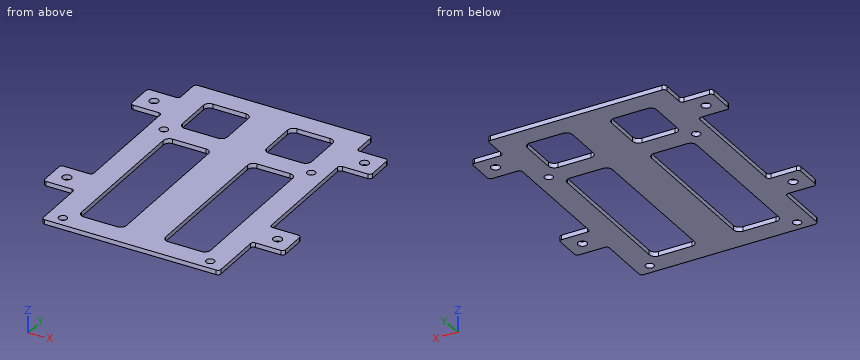
```python
from build123d import *

# Parameters (mm, degrees)
MODEL_R         = 1.375
MODEL_R_2       = 1.5
EXTRUDE_1_DEPTH = 1.5


with BuildPart() as part:
    # Model → Бобышка-Вытянуть1 (new body)
    with BuildSketch(Plane.XY):
        with BuildLine():
            ThreePointArc((-28.5, 7.535944945), (-29.207106781, 7.243051726), (-29.5, 6.535944945))
            Line((-29.5, 6.535944945), (-29.5, -0.464055055))
            ThreePointArc((-29.5, -0.464055055), (-29.792893219, -1.171161836), (-30.5, -1.464055055))
            Line((-30.5, -1.464055055), (-39, -1.464055055))
            ThreePointArc((-39, -1.464055055), (-39.707106781, -1.756948274), (-40, -2.464055055))
            Line((-40, -2.464055055), (-40, -10.464055055))
            ThreePointArc((-40, -10.464055055), (-39.707106781, -11.171161836), (-39, -11.464055055))
            Line((-39, -11.464055055), (-30.5, -11.464055055))
            ThreePointArc((-30.5, -11.464055055), (-29.792893219, -11.756948274), (-29.5, -12.464055055))
            Line((-29.5, -12.464055055), (-29.5, -50.464055055))
            ThreePointArc((-29.5, -50.464055055), (-29.792893219, -51.171161836), (-30.5, -51.464055055))
            Line((-30.5, -51.464055055), (-39, -51.464055055))
            ThreePointArc((-39, -51.464055055), (-39.707106781, -51.756948274), (-40, -52.464055055))
            Line((-40, -52.464055055), (-40, -60.464055055))
            ThreePointArc((-40, -60.464055055), (-39.707106781, -61.171161836), (-39, -61.464055055))
            Line((-39, -61.464055055), (-30.5, -61.464055055))
            ThreePointArc((-30.5, -61.464055055), (-29.792893219, -61.756948274), (-29.5, -62.464055055))
            Line((-29.5, -62.464055055), (-29.5, -79.464055055))
            ThreePointArc((-29.5, -79.464055055), (-29.207106781, -80.171161836), (-28.5, -80.464055055))
            Line((-28.5, -80.464055055), (28.5, -80.464055055))
            ThreePointArc((28.5, -80.464055055), (29.207106781, -80.171161836), (29.5, -79.464055055))
            Line((29.5, -79.464055055), (29.5, -62.464055055))
            ThreePointArc((29.5, -62.464055055), (29.792893219, -61.756948274), (30.5, -61.464055055))
            Line((30.5, -61.464055055), (39, -61.464055055))
            ThreePointArc((39, -61.464055055), (39.707106781, -61.171161836), (40, -60.464055055))
            Line((40, -60.464055055), (40, -52.464055055))
            ThreePointArc((40, -52.464055055), (39.707106781, -51.756948274), (39, -51.464055055))
            Line((39, -51.464055055), (30.5, -51.464055055))
            ThreePointArc((30.5, -51.464055055), (29.792893219, -51.171161836), (29.5, -50.464055055))
            Line((29.5, -50.464055055), (29.5, -12.464055055))
            ThreePointArc((29.5, -12.464055055), (29.792893219, -11.756948274), (30.5, -11.464055055))
            Line((30.5, -11.464055055), (39, -11.464055055))
            ThreePointArc((39, -11.464055055), (39.707106781, -11.171161836), (40, -10.464055055))
            Line((40, -10.464055055), (40, -2.464055055))
            ThreePointArc((40, -2.464055055), (39.707106781, -1.756948274), (39, -1.464055055))
            Line((39, -1.464055055), (30.5, -1.464055055))
            ThreePointArc((30.5, -1.464055055), (29.792893219, -1.171161836), (29.5, -0.464055055))
            Line((29.5, -0.464055055), (29.5, 6.535944945))
            ThreePointArc((29.5, 6.535944945), (29.207106781, 7.243051726), (28.5, 7.535944945))
            Line((28.5, 7.535944945), (-28.5, 7.535944945))
        make_face()
        with Locations((-24.5, -76.964055055)):
            Circle(MODEL_R, mode=Mode.SUBTRACT)
        with Locations((-35, -56.464055055)):
            Circle(MODEL_R_2, mode=Mode.SUBTRACT)
        with BuildLine():
            ThreePointArc((-21.5, -24.464055055), (-20.914213562, -23.049841493), (-19.5, -22.464055055))
            Line((-19.5, -22.464055055), (-8.5, -22.464055055))
            ThreePointArc((-8.5, -22.464055055), (-7.085786438, -23.049841493), (-6.5, -24.464055055))
            Line((-6.5, -24.464055055), (-6.5, -71.464055055))
            ThreePointArc((-6.5, -71.464055055), (-7.085786438, -72.878268617), (-8.5, -73.464055055))
            Line((-8.5, -73.464055055), (-19.5, -73.464055055))
            ThreePointArc((-19.5, -73.464055055), (-20.914213562, -72.878268617), (-21.5, -71.464055055))
            Line((-21.5, -71.464055055), (-21.5, -24.464055055))
        make_face(mode=Mode.SUBTRACT)
        with Locations((-24.5, -18.964055055)):
            Circle(MODEL_R, mode=Mode.SUBTRACT)
        with Locations((-35, -6.464055055)):
            Circle(MODEL_R_2, mode=Mode.SUBTRACT)
        with BuildLine():
            Line((-8.5, -15.464055055), (-19.5, -15.464055055))
            ThreePointArc((-19.5, -15.464055055), (-20.914213562, -14.878268617), (-21.5, -13.464055055))
            Line((-21.5, -13.464055055), (-21.5, -1.464055055))
            ThreePointArc((-21.5, -1.464055055), (-20.914213562, -0.049841493), (-19.5, 0.535944945))
            Line((-19.5, 0.535944945), (-8.5, 0.535944945))
            ThreePointArc((-8.5, 0.535944945), (-7.085786438, -0.049841493), (-6.5, -1.464055055))
            Line((-6.5, -1.464055055), (-6.5, -13.464055055))
            ThreePointArc((-6.5, -13.464055055), (-7.085786438, -14.878268617), (-8.5, -15.464055055))
        make_face(mode=Mode.SUBTRACT)
        with Locations((24.5, -76.964055055)):
            Circle(MODEL_R, mode=Mode.SUBTRACT)
        with BuildLine():
            Line((21.5, -24.464055055), (21.5, -71.464055055))
            ThreePointArc((21.5, -71.464055055), (20.914213562, -72.878268617), (19.5, -73.464055055))
            Line((19.5, -73.464055055), (8.5, -73.464055055))
            ThreePointArc((8.5, -73.464055055), (7.085786438, -72.878268617), (6.5, -71.464055055))
            Line((6.5, -71.464055055), (6.5, -24.464055055))
            ThreePointArc((6.5, -24.464055055), (7.085786438, -23.049841493), (8.5, -22.464055055))
            Line((8.5, -22.464055055), (19.5, -22.464055055))
            ThreePointArc((19.5, -22.464055055), (20.914213562, -23.049841493), (21.5, -24.464055055))
        make_face(mode=Mode.SUBTRACT)
        with Locations((35, -56.464055055)):
            Circle(MODEL_R_2, mode=Mode.SUBTRACT)
        with Locations((24.5, -18.964055055)):
            Circle(MODEL_R, mode=Mode.SUBTRACT)
        with BuildLine():
            ThreePointArc((21.5, -13.464055055), (20.914213562, -14.878268617), (19.5, -15.464055055))
            Line((19.5, -15.464055055), (8.5, -15.464055055))
            ThreePointArc((8.5, -15.464055055), (7.085786438, -14.878268617), (6.5, -13.464055055))
            Line((6.5, -13.464055055), (6.5, -1.464055055))
            ThreePointArc((6.5, -1.464055055), (7.085786438, -0.049841493), (8.5, 0.535944945))
            Line((8.5, 0.535944945), (19.5, 0.535944945))
            ThreePointArc((19.5, 0.535944945), (20.914213562, -0.049841493), (21.5, -1.464055055))
            Line((21.5, -1.464055055), (21.5, -13.464055055))
        make_face(mode=Mode.SUBTRACT)
        with Locations((35, -6.464055055)):
            Circle(MODEL_R_2, mode=Mode.SUBTRACT)
    extrude(amount=EXTRUDE_1_DEPTH)


solid = part.part
```
Geometry: final body of the model. Coordinates: model frame, mm. Round coordinates to 2 decimals unless told otherwise and drop trailing zeros. Write each loop counter-clockwise with the first axis right and the second up, starting at its lowest first coordinate (ties: lowest second). Pieces come first, ordered by that corner, then holes.
Item 1: Section query B-B (x = 12). Return loops of the section in (y, z).
Item 2: Pin query (flat end, axial travel): P1, Ø2.5, axis at x = 35, y = -6.46, coming from the -Z side; P2, Ø0.8, axis at x = -35.5, z = 1, coming from the +Y side. Return the tip coordinate at first contact, or that it passes through.
Item 3: Section query C-C (x = 35). Return loops of the section in (y, z).
Item 4: Section query A-A (y = -45.5). Return loops of the section in (x, z).
Item 5: Material intervals for L1, parallel to X at y = -2.5, z = 0.3; L2, parallel to Y at x = 24.5, z = 0.95; L3, parallel to Y at x = 19, z = 0.1, sorted ascending.
Item 6: Section query D-D (y = 2). Return loops of the section in (x, z).
Completed:
1. outline: (-80.46, 0) - (-73.46, 0) - (-73.46, 1.5) - (-80.46, 1.5) - close; (-22.46, 0) - (-15.46, 0) - (-15.46, 1.5) - (-22.46, 1.5) - close; (0.54, 0) - (7.54, 0) - (7.54, 1.5) - (0.54, 1.5) - close
2. P1: passes through
2. P2: stops at y = -1.46
3. outline: (-61.46, 0) - (-57.96, 0) - (-57.96, 1.5) - (-61.46, 1.5) - close; (-54.96, 0) - (-51.46, 0) - (-51.46, 1.5) - (-54.96, 1.5) - close; (-11.46, 0) - (-7.96, 0) - (-7.96, 1.5) - (-11.46, 1.5) - close; (-4.96, 0) - (-1.46, 0) - (-1.46, 1.5) - (-4.96, 1.5) - close
4. outline: (-29.5, 0) - (-21.5, 0) - (-21.5, 1.5) - (-29.5, 1.5) - close; (-6.5, 0) - (6.5, 0) - (6.5, 1.5) - (-6.5, 1.5) - close; (21.5, 0) - (29.5, 0) - (29.5, 1.5) - (21.5, 1.5) - close
5. L1: x = -40 to -21.5, -6.5 to 6.5, 21.5 to 40
5. L2: y = -80.46 to -78.34, -75.59 to -20.34, -17.59 to 7.54
5. L3: y = -80.46 to -73.46, -22.46 to -15.46, 0.54 to 7.54
6. outline: (-29.5, 0) - (29.5, 0) - (29.5, 1.5) - (-29.5, 1.5) - close
